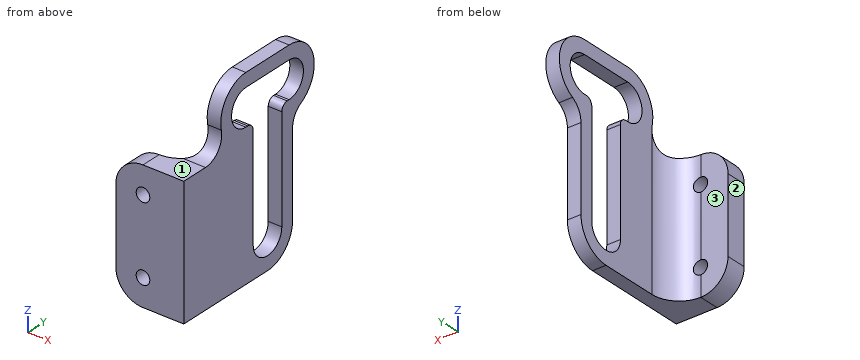
from build123d import *

# Parameters (mm, degrees)
BOSS_EXTRUDE1_DEPTH = 2
BOSS_EXTRUDE2_START = -16
BOSS_EXTRUDE2_DEPTH = 2
SKETCH3_W           = 19.045654227
SKETCH3_H           = 3
BOSS_EXTRUDE3_DEPTH = 8
FILLET1_R           = 4
SKETCH5_W           = 1
SKETCH5_H           = 3
HOLE1_AT_2_COUNT    = 2
HOLE1_AT_2_PITCH    = 11.045654227
CUT_EXTRUDE1_START  = 2
SKETCH6_R           = 1
CUT_EXTRUDE1_DEPTH  = 2
FILLET2_R           = 3
FILLET3_R           = 3


# Read off the part's stored shape, not the designer's step: Boss-Extrude2
with BuildPart() as part:
    # Sketch1 → Boss-Extrude1 (new body)
    with BuildSketch(Plane.ZY.offset(14)):
        with BuildLine():
            Line((12.895654227, 10.15), (-1.5, 10.15))
            ThreePointArc((-1.5, 10.15), (-6.15, 5.5), (-1.5, 0.85))
            Line((-1.5, 0.85), (12.895654227, 0.85))
            ThreePointArc((12.895654227, 0.85), (17.825800671, -3.138572401), (22.15, 1.5))
            Line((22.15, 1.5), (22.15, 9.5))
            ThreePointArc((22.15, 9.5), (17.825800671, 14.138572401), (12.895654227, 10.15))
        make_face()
        with BuildLine():
            Line((13.85, 8.15), (-1.5, 8.15))
            ThreePointArc((-1.5, 8.15), (-4.15, 5.5), (-1.5, 2.85))
            Line((-1.5, 2.85), (13.85, 2.85))
            ThreePointArc((13.85, 2.85), (14.557106781, 2.557106781), (14.85, 1.85))
            Line((14.85, 1.85), (14.85, 1.5))
            ThreePointArc((14.85, 1.5), (17.5, -1.15), (20.15, 1.5))
            Line((20.15, 1.5), (20.15, 9.5))
            ThreePointArc((20.15, 9.5), (17.5, 12.15), (14.85, 9.5))
            Line((14.85, 9.5), (14.85, 9.15))
            ThreePointArc((14.85, 9.15), (14.557106781, 8.442893219), (13.85, 8.15))
        make_face(mode=Mode.SUBTRACT)
    extrude(amount=BOSS_EXTRUDE1_DEPTH)

    # Boss-Extrude2 outline → Boss-Extrude2 (add)
    with BuildSketch(Plane.YZ.offset(BOSS_EXTRUDE2_START)):
        with BuildLine():
            Line((-10, 12.895654227), (-10, -6.15))
            Line((-10, -6.15), (5.5, -6.15))
            ThreePointArc((5.5, -6.15), (2.211953467, -4.788046533), (0.85, -1.5))
            Line((0.85, -1.5), (0.85, 12.895654227))
            Line((0.85, 12.895654227), (-10, 12.895654227))
        make_face()
    extrude(amount=BOSS_EXTRUDE2_DEPTH)

    # Sketch3 → Boss-Extrude3 (add)
    with BuildSketch(Plane.ZY.offset(16)):
        with Locations((3.372827114, -8.5)):
            Rectangle(SKETCH3_W, SKETCH3_H)
    extrude(amount=BOSS_EXTRUDE3_DEPTH)

    # Fillet1
    fillet1_edges = [part.edges().sort_by_distance(p)[0] for p in [
        (-24, -8.5, 12.895654227),
        (-24, -8.5, -6.15),
        (-16, -7, 3.372827113),
    ]]
    fillet(fillet1_edges, radius=FILLET1_R - 0.0001)  # a hair under: the kernel refuses the full size

    # Sketch5 → Hole1 (revolve, cut)
    with BuildSketch(Plane(origin=(-20, -7, -2.15), x_dir=(0, 0, 1), z_dir=(1, 0, 0))):
        with Locations((0.5, 1.5)):
            Rectangle(SKETCH5_W, SKETCH5_H)
    hole1 = revolve(axis=Axis((-20, -117, -2.15), (0, 1, 0)), mode=Mode.SUBTRACT)

    # Hole1 at 2: Hole1 ×2
    with Locations(*[(0, 0, i * HOLE1_AT_2_PITCH) for i in range(1, HOLE1_AT_2_COUNT)]):
        add(hole1, mode=Mode.SUBTRACT)

    # Sketch6 → Cut-Extrude1 (cut)
    with BuildSketch(Plane(origin=(0, -7, 0), x_dir=(1, 0, 0), z_dir=(0, 1, 0)).offset(CUT_EXTRUDE1_START)):
        with Locations(Location((-20, -8.895654227, 0), (0, 0, 270))):
            Circle(SKETCH6_R)
        with Locations(Location((-20, 2.15, 0), (0, 0, 270))):
            Circle(SKETCH6_R)
    extrude(amount=-CUT_EXTRUDE1_DEPTH, mode=Mode.SUBTRACT)

    # Fillet2
    fillet2_edges = [part.edges().sort_by_distance(p)[0] for p in [
        (-15, 10.15, 12.895654227),
    ]]
    fillet(fillet2_edges, radius=FILLET2_R)

    # Fillet3
    fillet3_edges = [part.edges().sort_by_distance(p)[0] for p in [
        (-15, 0.85, 12.895654227),
    ]]
    fillet(fillet3_edges, radius=FILLET3_R)


solid = part.part
Input: part model. Units: mm. Frame: model coordinates. Face numbers are marked on the shaded views. A direction names the side the tool comes from. Coordinates: 2 decimals unless noted, no trailing zeros. Order: outer loops, then holes, each group sorted by start corner. A loop starts at its lowest first (then second) coordinate and runs counter-clockwise, first axis right, second up.
1. Cut plane C-C, the plane x = -14.75. Return loops of the section in (y, z).
Checked values:
outline: (-10, -6.15) - (5.5, -6.15) arc R4.65 ccw to (10.15, -1.5) - (10.15, 10.78) arc R3 cw to (11.72, 13.41) arc R4.65 ccw to (9.5, 22.15) - (1.5, 22.15) arc R4.65 ccw to (-3.05, 16.52) arc R3 cw to (-5.98, 12.9) - (-10, 12.9) - close; hole (1.5, 14.85) - (1.85, 14.85) arc R1 cw to (2.85, 13.85) - (2.85, -1.5) arc R2.65 ccw to (8.15, -1.5) - (8.15, 13.85) arc R1 cw to (9.15, 14.85) - (9.5, 14.85) arc R2.65 ccw to (9.5, 20.15) - (1.5, 20.15) arc R2.65 ccw to start
2. Cut plane A-A, the plane z = 17.5. Return loops of the section in (x, y).
Checked values:
outline: (-16, -3.15) - (-14, -3.15) - (-14, -1.15) - (-16, -1.15) - close; (-16, 12.15) - (-14, 12.15) - (-14, 14.15) - (-16, 14.15) - close
3. Cut plane B-B, the plane y = 4.75. Return loops of the section in (x, z).
Checked values:
outline: (-16, -6.15) - (-14, -6.15) - (-14, -4.04) - (-16, -4.04) - close; (-16, 20.15) - (-14, 20.15) - (-14, 22.15) - (-16, 22.15) - close
4. Access query for the marked faces 1, 2 and 3. Directions: +Z, -Z, +X, -X, +Y, -Y. A direction counts if a zero-diameter tool reaches every point of the face in a straight line with its end or side. Return the directions, or none.
Checked values:
face 1: +Z, +X, -X, -Y
face 2: +Z, -Z, -X, +Y, -Y
face 3: +Z, -Z, -X, +Y
5. Cut plane D-D, the plane z = 2.25. Return loops of the section in (x, y).
Checked values:
outline: (-24, -10) - (-14, -10) - (-14, 2.85) - (-16, 2.85) - (-16, -3) arc R4 cw to (-20, -7) - (-24, -7) - close; (-16, 8.15) - (-14, 8.15) - (-14, 10.15) - (-16, 10.15) - close
6. Ray query, line 1 along Z through (x, y) = (-20, -8.5); line 2 along X through (y, z) = (-8.65, -2.15); line 3 along Y through (x, z) = (-15, -1). Return the intervals inside material, ascending.
Checked values:
line 1: z = -6.15 to -3.15, -1.15 to 7.9, 9.9 to 12.9
line 2: x = -24 to -21, -19 to -14
line 3: y = -10 to 2.85, 8.15 to 10.15
7. Contact query for flat-ended pins moving along their axis: P1, Ø1, axis at x = -15.5, z = 8.5, coming from the +Y side; P2, Ø3, axis at x = -20.5, z = 1.5, coming from the +Y side; P3, Ø1, axis at x = -15, y = 7.5, coming from the -Z side; P4, Ø1.5, axis at x = -16.5, y = 9.5, coming from the +Z side. Output: stop coordinate, or through.
Checked values:
P1: stops at y = 10.15
P2: stops at y = -6.87
P3: stops at z = -5.9
P4: stops at z = 22.15
